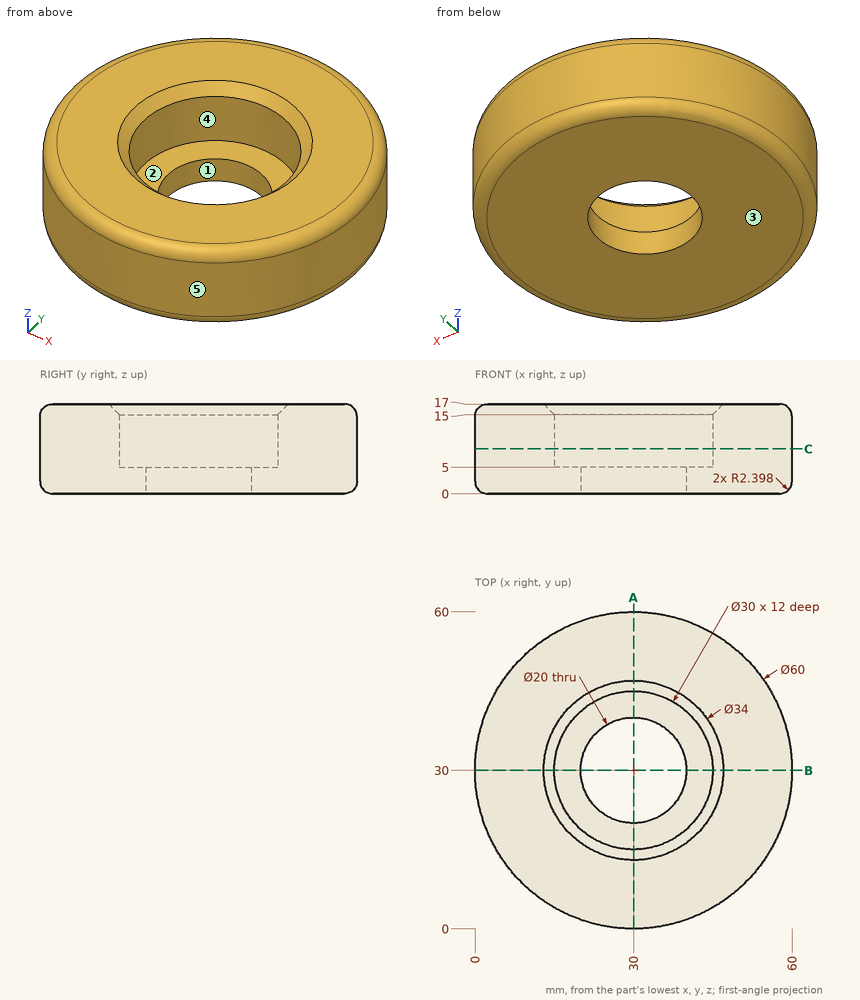
Design review of the part shown in the three views and the two pictorial views. Dimensions are in mm from the part's minimum x, y and z. A direction names the side the tool comes from. Give positions to 0.01 mm unless a question says otherwise; leave off trailing zeros. Order: outer loops, then holes, each group sorted by start corner. A loop starts at its lowest first (then second) coordinate and runs counter-clockwise, first axis right, second up. Notation, with made-up numbers: (-28, 1) -> (17, 1) arc R24 ccw to (17, 28) -> close; hole circle Ø2 at (57.5, 88). An arc over 180 degrees is marked (long way). Write each question's results on one line, items separated by ' | '. Start each with the question number.
Q1. Machinability: for the marked faces 1 and 2, which of the approach directions +Z, -Z, +X, -X, +Y, -Y give a long, thin tool a straight path to every point of the face, cutting with its end or side? Answer none if there is none.
Q2. Add section A-A on x = 30. Give the boundary of the cut face in (y, z), and give its area (3 significant figures).
Q3. Wall thickness on L1, parallel to X at y = 30, z = 9.25; L2, parallel to Y at x = 30, z = 3.85: over which ranges is each line inside the solid? List them lowest first. Write a range as from..to.
Q4. For pin 1 (1 mm diameter, centred on x = 28, y = 45.5, fed in from +Z); pin 2 (10 mm diameter, centred on y = 10.5, z = 3, fed in from +X); pin 3 (10 mm diameter, centred on x = 48, z = 12.5, fed in from +Y); pin 4 (12 mm diameter, centred on x = 30, y = 30, fed in from -Z), all flat-tipped, find the tip position at first contact; note any pin that passes through.
Q5. Mouldability with a two-part tool opening along Y and no side actions: class the marked faces 3, 4 and 5 as +Y half, -Y half, draft (parallel to the pull), parting line (faces both ways), or undercut.
Q6. Add section C-C on z = 8.5. Give the boundary of the cut face in (x, y).
Found:
1) face 1: +Z, -Z | face 2: +Z
2) outline: (0, 2.4) arc R2.4 ccw to (2.4, 0) -> (20, 0) -> (20, 5) -> (15, 5) -> (15, 15) -> (13, 17) -> (2.4, 17) arc R2.4 ccw to (0, 14.6) -> close; (40, 0) -> (57.6, 0) arc R2.4 ccw to (60, 2.4) -> (60, 14.6) arc R2.4 ccw to (57.6, 17) -> (47, 17) -> (45, 15) -> (45, 5) -> (40, 5) -> close | area: 551 mm2
3) L1: x = 0..15, 45..60 | L2: y = 0..20, 40..60
4) pin 1: stops at z = 16.13 | pin 2: stops at x = 56.26 | pin 3: stops at y = 57.04 | pin 4: passes through
5) face 3: draft | face 4: undercut | face 5: parting line
6) outline: circle Ø60 at (30, 30); hole circle Ø30 at (30, 30)
